Verification items for the finished model (mm, model axes). A direction names the side the tool comes from. Coordinates: 2 decimals unless noted, no trailing zeros. Write each loop counter-clockwise with the first axis right and the second up, starting at its lowest first coordinate (ties: lowest second). Pieces come first, ordered by that corner, then holes. Notation, with made-up numbers: (81.5, -26) - (108.5, -26) arc R18 cw to (108.5, -8) - close; hole circle Ø4 at (5.25, 10.5). An arc over 180 degrees is marked (long way). Use one line per item in the form item = value. Start each with the question number.
(1) Gauge pin test, flat ends, axial feed: pin 1 Ø1 at (y, z) = (26, 3.5) entering from -X; pin 2 Ø15.5 at (y, z) = (7.5, -13) entering from +X; pin 3 Ø8 at (x, y) = (39.5, 15) entering from +Z. Record the tip position at first contact, or that the pin passes through.
(2) Material ranges on line 1 (Z direction, x = 29, y = 17); line 2 (Y direction, x = 38, z = 2.5) (3 decimals); line 3 (X direction, y = 15, z = -2.5), recorded low to high. Write a range as [from, to].
(3) Sectioned sample at C-C (z = -1). Record the cut outline in (x, y) (3 decimals), and give its area (3 significant figures).
(4) Mould release check, pull along X, two halves, no side actions. Record for faces 6 (the cylindrical face through (0, 27, -31)), 7 (the flat face through (39, 27, -37.427)), 8 (the cylindrical face through (76.274, 27.187, -12.013)): released by +X, released by -X, zero draft, split by the parting line, or undercut.
(5) Sectioned sample at D-D (z = -25.5). Record the cut outline in (x, y) (3 decimals), and give its area (3 significant figures).
(6) Sectioned sample at B-B (y = 31). Record the cut outline in (x, z), and give its area (3 significant figures).
(7) Sectioned sample at A-A (x = 58). Record the cut outline in (y, z) (3 decimals), and give its area (3 significant figures).
(8) Tool access check on faces 1 (the flat face through (34, 34.925, -13)), 2 (the flat face through (2, 33, 0)), 3 (the cylindrical face through (0, 27, 6)), 4 (the flat face through (60.376, 9, -12)), 5 (the flat face through (2, 33, -24.714)). Record the directions out of +Z, -Z, +X, -X, +Y, -Y that give a thin tool (end or side, any length) a straight path to the whole face; none if there is none.
from build123d import *

# Parameters (mm, degrees)
SKETCH1_W                = 60.3758
SKETCH1_H                = 24.7142
BOSS_EXTRUDE1_DEPTH      = 34.925
BOSS_EXTRUDE2_DEPTH      = 12.7
BOSS_EXTRUDE2_DEPTH_BACK = 37.4269


with BuildPart() as part:
    # Sketch1 → Boss-Extrude1 (new body)
    with BuildSketch(Plane(origin=(0, 0, 0), x_dir=(1, 0, 0), z_dir=(0, 1, 0))):
        with Locations((30.1879, 12.3571)):
            Rectangle(SKETCH1_W, SKETCH1_H)
    extrude(amount=BOSS_EXTRUDE1_DEPTH)

    # Sketch2 → Boss-Extrude2 (add, two sides)
    with BuildSketch(Plane.XY) as boss_extrude2_sk:
        with BuildLine():
            Line((7.9121, 34.925), (68.3641, 34.925))
            ThreePointArc((68.3641, 34.925), (76.2762, 27.0129), (68.3641, 19.1008))
            Line((68.3641, 19.1008), (7.9121, 19.1008))
            ThreePointArc((7.9121, 19.1008), (0, 27.0129), (7.9121, 34.925))
        make_face()
    extrude(amount=BOSS_EXTRUDE2_DEPTH)
    extrude(boss_extrude2_sk.sketch, amount=-BOSS_EXTRUDE2_DEPTH_BACK)


solid = part.part
Answers below:
q1.pin_1 = 0.02
q1.pin_2 = 60.38
q1.pin_3 = 0
q2.line_1 = [-24.71, 0]
q2.line_2 = [19.101, 34.925]
q2.line_3 = [0, 60.38]
q3.outline = (0, 0) - (60.376, 0) - (60.376, 19.101) - (68.364, 19.101) arc R7.912 ccw to (68.364, 34.925) - (0, 34.925) - close
q3.area = 2,330 mm2
q4.face_6 = released by -X
q4.face_7 = zero draft
q4.face_8 = released by +X
q5.outline = (7.912, 19.101) - (68.364, 19.101) arc R7.912 ccw to (68.364, 34.925) - (7.912, 34.925) arc R7.912 ccw to start
q5.area = 1,150 mm2
q6.outline = (0, -24.71) - (1.08, -24.71) - (1.08, -37.43) - (75.2, -37.43) - (75.2, 12.7) - (1.08, 12.7) - (1.08, 0) - (0, 0) - close
q6.area = 3,740 mm2
q7.outline = (0, -24.714) - (19.101, -24.714) - (19.101, -37.427) - (34.925, -37.427) - (34.925, 12.7) - (19.101, 12.7) - (19.101, 0) - (0, 0) - close
q7.area = 1,270 mm2
q8.face_1 = +Z, -Z, +X, -X, +Y
q8.face_2 = +Z, -X, +Y
q8.face_3 = +Z, -X
q8.face_4 = +Z, -Z, +X, -Y
q8.face_5 = -Z, -X, +Y
